Geometry check sheet. Reference: the model listing, model coordinates, mm. A direction names the side the tool comes from. Round coordinates to 2 decimals unless told otherwise and drop trailing zeros. Loops run counter-clockwise (first coordinate to the right, second up) from the corner with the lowest first, then second, coordinate; pieces in that order, holes last. Notation, with made-up numbers: (-34.5, -37.5) -> (20.5, -37.5) arc R15 cw to (20.5, -20.5) -> close; hole circle Ø11 at (76.25, 38). An arc over 180 degrees is marked (long way). Use a Markdown table: item, result. Add a question column.
Q1. Sectioned sample at D-D, the plane z = 6.25. Enter the section's corners in (x, y), then the cut area to 3 significant figures.
Q2. Gauge pin test, flat ends, axial feed: P1, Ø1, axis at y = 58.5, z = 10.5, coming from the -X side; P2, Ø5, axis at x = -66, y = 63, coming from the +Z side; P3, Ø3, axis at x = -46.32, y = 61.98, coming from the +Z side; P4, Ø3, axis at y = 62, z = 13.5, coming from the +X side. Record the tip position at first contact, or that the pin passes through.
Q3. Sectioned sample at C-C, the plane y = 59.5. Enter the section's corners in (x, z), then the cut area to 3 significant figures.
Q4. Sectioned sample at A-A, the plane x = -57.5. Enter the section's corners in (y, z), then the cut area to 3 significant figures.
Q5. Set-up check for faces 1 (the face through (-70.03, 62.05, 3)), 2 (the face through (-60.124, 62, 13)), 3 (the face through (-71.624, 62, 1)), 4 (the face through (-63.524, 62.959, 2.014)), 5 (the face through (-51.324, 62, 14)): record each of +Z, -Z, +X, -X, +Y, -Y from which the full face is reachable in a straight line by a thin tool's end or side.
Q6. Release check for a two-part mould opening along X. For faces 6 (the face through (-65.1, 61.35, 0.49)), 7 (the face through (-61.624, 62, 14)), 8 (the face through (-50, 62, 3)) record: released by +X, released by -X, zero draft, split by the parting line, or undercut.
Q7. Sectioned sample at B-B, the plane y = 61.5. Enter the section's corners in (x, z).
Q8. Material ranges on L1, parallel to Y at x = -53.5, z = 7; L2, parallel to X at y = 59.5, z = 19; L3, parallel to Z at x = -43.5, y = 59.25, recorded low to high.
```python
from build123d import *

# Parameters (mm, degrees)
CROQUIS1_W              = 10.3
CROQUIS1_H              = 10.3
CROQUIS1_W_2            = 7.3
CROQUIS1_H_2            = 7.3
SALIENTE_EXTRUIR1_DEPTH = 26
CROQUIS2_W              = 10
CROQUIS2_H              = 10.3
CROQUIS2_R              = 1.65
SALIENTE_EXTRUIR2_DEPTH = 3
CROQUIS3_R              = 3.25
CORTAR_EXTRUIR1_DEPTH   = 2


with BuildPart() as part:
    # Croquis1 → Saliente-Extruir1 (new body)
    with BuildSketch(Plane.XY):
        with Locations((-56.473903104, 61.98267988)):
            Rectangle(CROQUIS1_W, CROQUIS1_H)
        with Locations((-56.473903104, 61.98267988)):
            Rectangle(CROQUIS1_W_2, CROQUIS1_H_2, mode=Mode.SUBTRACT)
    extrude(amount=SALIENTE_EXTRUIR1_DEPTH)

    # Croquis2 → Saliente-Extruir2 (add)
    with BuildSketch(Plane.XY):
        with Locations((-46.323903104, 61.98267988)):
            Rectangle(CROQUIS2_W, CROQUIS2_H)
        with Locations((-46.323903104, 61.98267988)):
            Circle(CROQUIS2_R, mode=Mode.SUBTRACT)
        with Locations((-66.623903104, 61.98267988)):
            Rectangle(CROQUIS2_W, CROQUIS2_H)
        with Locations((-66.623903104, 61.98267988)):
            Circle(CROQUIS2_R, mode=Mode.SUBTRACT)
    extrude(amount=SALIENTE_EXTRUIR2_DEPTH)

    # Croquis3 → Cortar-Extruir1 (cut)
    with BuildSketch(Plane.XY.offset(3)):
        with Locations((-66.623903104, 61.98267988)):
            Circle(CROQUIS3_R)
        with Locations((-46.323903104, 61.98267988)):
            Circle(CROQUIS3_R)
    extrude(amount=-CORTAR_EXTRUIR1_DEPTH, mode=Mode.SUBTRACT)


solid = part.part
```
Values:
| question | item | result |
|---|---|---|
| 1 | outline | (-61.62, 56.83) -> (-51.32, 56.83) -> (-51.32, 67.13) -> (-61.62, 67.13) -> close; hole (-60.12, 58.33) -> (-52.82, 58.33) -> (-52.82, 65.63) -> (-60.12, 65.63) -> close |
| 1 | area | 52.8 mm^2 |
| 2 | P1 | x = -61.62 |
| 2 | P2 | z = 3 |
| 2 | P3 | through |
| 2 | P4 | x = -51.32 |
| 3 | outline | (-71.62, 0) -> (-60.12, 0) -> (-60.12, 26) -> (-61.62, 26) -> (-61.62, 3) -> (-64.53, 3) -> (-64.53, 1) -> (-68.72, 1) -> (-68.72, 3) -> (-71.62, 3) -> close; (-52.82, 0) -> (-41.32, 0) -> (-41.32, 3) -> (-44.23, 3) -> (-44.23, 1) -> (-48.42, 1) -> (-48.42, 3) -> (-51.32, 3) -> (-51.32, 26) -> (-52.82, 26) -> close |
| 3 | area | 121 mm^2 |
| 4 | outline | (56.83, 0) -> (58.33, 0) -> (58.33, 26) -> (56.83, 26) -> close; (65.63, 0) -> (67.13, 0) -> (67.13, 26) -> (65.63, 26) -> close |
| 4 | area | 78.0 mm^2 |
| 5 | face 1 | +Z, -X, +Y, -Y |
| 5 | face 2 | +Z, -Z |
| 5 | face 3 | +Z, -Z, -X, +Y, -Y |
| 5 | face 4 | +Z |
| 5 | face 5 | +Z, +X, +Y, -Y |
| 6 | face 6 | undercut |
| 6 | face 7 | released by -X |
| 6 | face 8 | zero draft |
| 7 | outline | (-71.62, 0) -> (-68.2, 0) -> (-68.2, 1) -> (-69.84, 1) -> (-69.84, 3) -> (-71.62, 3) -> close; (-65.05, 0) -> (-60.12, 0) -> (-60.12, 26) -> (-61.62, 26) -> (-61.62, 3) -> (-63.41, 3) -> (-63.41, 1) -> (-65.05, 1) -> close; (-52.82, 0) -> (-47.9, 0) -> (-47.9, 1) -> (-49.54, 1) -> (-49.54, 3) -> (-51.32, 3) -> (-51.32, 26) -> (-52.82, 26) -> close; (-44.75, 0) -> (-41.32, 0) -> (-41.32, 3) -> (-43.11, 3) -> (-43.11, 1) -> (-44.75, 1) -> close |
| 8 | L1 | 56.83 to 58.33, 65.63 to 67.13 |
| 8 | L2 | -61.62 to -60.12, -52.82 to -51.32 |
| 8 | L3 | 0 to 3 |
